Design review of the part built by this model. Coordinates are the model's own, in mm. A direction names the side the tool comes from. Coordinates: 2 decimals unless noted, no trailing zeros. Loops run counter-clockwise (first coordinate to the right, second up) from the corner with the lowest first, then second, coordinate; pieces in that order, holes last. Notation, with made-up numbers: (6.25, 80.5) -> (12.25, 80.5) arc R20 cw to (12.25, 102.5) -> close; hole circle Ø8 at (-0.75, 82.5). An arc over 180 degrees is marked (long way). Answer in a Markdown table with one row per item.
```python
from build123d import *

# Parameters (mm, degrees)
SKETCH3_W           = 15.24
SKETCH3_H           = 63.5
FILLET5_R           = 5.08
SHELL5_T            = -1.27
SKETCH9_R           = 13.97
SKETCH9_R_2         = 12.7
BOSS_EXTRUDE5_DEPTH = 1.27


with BuildPart() as part:
    # Sketch3 → Revolve1 (revolve)
    with BuildSketch(Plane(origin=(0, 0, 0), x_dir=(0, 0, -1), z_dir=(1, 0, 0))):
        with Locations((7.62, 31.75)):
            Rectangle(SKETCH3_W, SKETCH3_H)
    revolve(axis=Axis((0, 0, 0), (0, 1, 0)))

    # Fillet5
    fillet5_edges = [part.edges().sort_by_distance(p)[0] for p in [
        (0, 0, 15.24),
    ]]
    fillet(fillet5_edges, radius=FILLET5_R)

    # Shell5
    shell5_openings = [part.faces().sort_by_distance(p)[0] for p in [
        (0, 63.5, 0),
    ]]
    offset(amount=SHELL5_T, openings=shell5_openings, kind=Kind.INTERSECTION)

    # Sketch9 → Boss-Extrude5 (add)
    with BuildSketch(Plane(origin=(0, 63.5, 0), x_dir=(1, 0, 0), z_dir=(0, 1, 0))):
        with Locations(Location((0, 0, 0), (0, 0, 90))):
            Circle(SKETCH9_R)
        with Locations(Location((0, 0, 0), (0, 0, 270))):
            Circle(SKETCH9_R_2, mode=Mode.SUBTRACT)
    extrude(amount=-BOSS_EXTRUDE5_DEPTH)


solid = part.part
```
(1) Take a section at A-A on z = 0. Give the boundary of the cut face in (x, y), and give its area (3 significant figures).
Evaluation:
| item | result |
|---|---|
| outline | (-15.24, 5.08) arc R5.08 ccw to (-10.16, 0) -> (10.16, 0) arc R5.08 ccw to (15.24, 5.08) -> (15.24, 63.5) -> (12.7, 63.5) -> (12.7, 62.23) -> (13.97, 62.23) -> (13.97, 5.08) arc R3.81 cw to (10.16, 1.27) -> (-10.16, 1.27) arc R3.81 cw to (-13.97, 5.08) -> (-13.97, 62.23) -> (-12.7, 62.23) -> (-12.7, 63.5) -> (-15.24, 63.5) -> close |
| area | 195 mm² |
(2) For pin 1 (3 mm diameter, centred on x = -3, y = 54, fed in from +Z); pin 2 (6 mm diameter, centred on x = -2.5, z = 6, fed in from +Y); pin 3 (10 mm diameter, centred on x = 10.5, y = 47.5, fed in from -Z), all flat-tipped, find the tip position at first contact; note any pin that passes through.
Evaluation:
| item | result |
|---|---|
| pin 1 | stops at z = 15.17 |
| pin 2 | stops at y = 1.27 |
| pin 3 | stops at z = -14.21 |
(3) Take a section at C-C on y = 47. Give the boundary of the cut face in (x, z), and give its area (3 significant figures).
Evaluation:
| item | result |
|---|---|
| outline | circle Ø30.48 at (0, 0); hole circle Ø27.94 at (0, 0) |
| area | 117 mm² |
(4) Draft analysis for pull direction Y (two halves, no side actions). For faces 4 (the flat face through (11.32, 62.23, -6.14)), 5 (the cylindrical face through (14.88, 34.7, 3.3)), 6 (the flat face through (0, 0, 0)), state which applies: pulls with the +Y half, pulls with the -Y half, needs draft (parallel to the pull), parting line crosses it, or undercut.
Evaluation:
| item | result |
|---|---|
| face 4 | undercut |
| face 5 | needs draft |
| face 6 | pulls with the -Y half |
(5) To check wall thickness, follow probe 1 along Z at (x, y) = (0, 50.5); probe 2 along X at (y, z) = (62.75, 0); probe 3 along X at (y, z) = (15, -0.5). State the ranges of each line that lie inside material, in increasing order.
Evaluation:
| item | result |
|---|---|
| probe 1 | z = -15.24 to -13.97, 13.97 to 15.24 |
| probe 2 | x = -15.24 to -12.7, 12.7 to 15.24 |
| probe 3 | x = -15.23 to -13.96, 13.96 to 15.23 |
(6) Tool access review of faces 1 (the flat face through (0, 1.27, 0)), 2 (the cylindrical face through (-13.85, 34.06, 1.82)), 3 (the flat face through (-12.5, 63.5, 3.5)): name each direction out of +Z, -Z, +X, -X, +Y, -Y from which nothing blocks a thin tool from reaching the whole face with its end or side.
Evaluation:
| item | result |
|---|---|
| face 1 | +Y |
| face 2 | none |
| face 3 | +Z, -Z, +X, -X, +Y |
(7) Take a section at B-B on x = 0. Give the boundary of the cut face in (y, z).
Evaluation:
| item | result |
|---|---|
| outline | (0, -10.16) arc R5.08 ccw to (5.08, -15.24) -> (63.5, -15.24) -> (63.5, -12.7) -> (62.23, -12.7) -> (62.23, -13.97) -> (5.08, -13.97) arc R3.81 cw to (1.27, -10.16) -> (1.27, 10.16) arc R3.81 cw to (5.08, 13.97) -> (62.23, 13.97) -> (62.23, 12.7) -> (63.5, 12.7) -> (63.5, 15.24) -> (5.08, 15.24) arc R5.08 ccw to (0, 10.16) -> close |
